Could you check a few things on this model? Use its own coordinates, in mm. A direction names the side the tool comes from. Coordinates: 2 decimals unless noted, no trailing zeros. Order: outer loops, then holes, each group sorted by start corner. A loop starts at its lowest first (then second) coordinate and runs counter-clockwise, first axis right, second up. Notation, with made-up numbers: M 48,17.25 L 74,17.25 A30 cw 74,43.25 Z; hole C 68.5,32.5 d8. An arc over 180 degrees is marked long. Put each result on its own line as item: value. Start each with the question number.
```python
from build123d import *

# Parameters (mm, degrees)
BOSS_EXTRUDE1_DEPTH = 5


with BuildPart() as part:
    # Sketch1 → Boss-Extrude1 (new body)
    with BuildSketch(Plane.XY):
        Polygon((25, 127.5), (20, 127.5), (20, 147.5), (25, 147.5), (25, 165), (32.5, 165), (32.5, 170), (47.5, 170), (47.5, 165), (55, 165), (55, 40), (47.5, 40), (47.5, 35), (32.5, 35), (32.5, 40), (25, 40), (25, 57.5), (20, 57.5), (20, 77.5), (25, 77.5), (25, 92.5), (20, 92.5), (20, 112.5), (25, 112.5), align=None)
    extrude(amount=-BOSS_EXTRUDE1_DEPTH)


solid = part.part
```
Item 1: For faces 5 (the flat face through (25, 85, -2)), 6 (the flat face through (25, 49, -2)), 7 (the flat face through (32.5, 167, -2)), 8 (the flat face through (47.5, 168, -2)), which set-ups out of +Z, -Z, +X, -X, +Y, -Y let a thin tool reach every point of the face, with its end or its side?
Item 2: If we section it at C-C on x = 52: Write out the boundary of the cut face in (y, z), then the cut area to 3 significant figures.
Item 3: If we section it at A-A on x = 23: Write out the boundary of the cut face in (y, z), then the cut area to 3 significant figures.
Item 4: I need wall thicknesses on probe 1 along X at (y, z) = (114, -1.2); probe 2 along Y at (x, z) = (53.5, -4.55). Which ranges of each line are inside material? Lowest first, please.
Item 5: If we section it at D-D on y = 79: Write out the boundary of the cut face in (x, z).
Item 6: For pin 1 Ø2.5 at (y, z) = (46, -3) entering from -X; pin 2 Ø1.5 at (y, z) = (38.5, -3) entering from -X; pin 3 Ø2.5 at (x, z) = (23, -2) entering from +Y; pin 4 Ø2 at (x, y) = (26, 123) entering from +Z, each with a flat end and sliding along its axis, tell me the tip position at first contact or that it passes through.
Item 7: If we mould it in two halves opening along Y, with no side actions, what happens to faces 1 (the flat face through (38, 103, -5)), 2 (the flat face through (29, 165, -2)), 3 (the flat face through (40, 35, -2)), 4 (the flat face through (22, 112.5, -2))? For each: released by +Y, released by -Y, zero draft, split by the parting line, or undercut.
Item 8: If we section it at B-B on z = -1.7: Write out the boundary of the cut face in (x, y).
Geometry check:
1. face 5: +Z, -Z, -X
1. face 6: +Z, -Z, -X, -Y
1. face 7: +Z, -Z, -X, +Y
1. face 8: +Z, -Z, +X, +Y
2. outline: M 40,-5 L 165,-5 L 165,0 L 40,0 Z
2. area: 625 mm²
3. outline: M 57.5,-5 L 77.5,-5 L 77.5,0 L 57.5,0 Z; M 92.5,-5 L 112.5,-5 L 112.5,0 L 92.5,0 Z; M 127.5,-5 L 147.5,-5 L 147.5,0 L 127.5,0 Z
3. area: 300 mm²
4. probe 1: x = 25 to 55
4. probe 2: y = 40 to 165
5. outline: M 25,-5 L 55,-5 L 55,0 L 25,0 Z
6. pin 1: stops at x = 25
6. pin 2: stops at x = 32.5
6. pin 3: stops at y = 147.5
6. pin 4: stops at z = 0
7. face 1: zero draft
7. face 2: released by +Y
7. face 3: released by -Y
7. face 4: undercut
8. outline: M 20,57.5 L 25,57.5 L 25,40 L 32.5,40 L 32.5,35 L 47.5,35 L 47.5,40 L 55,40 L 55,165 L 47.5,165 L 47.5,170 L 32.5,170 L 32.5,165 L 25,165 L 25,147.5 L 20,147.5 L 20,127.5 L 25,127.5 L 25,112.5 L 20,112.5 L 20,92.5 L 25,92.5 L 25,77.5 L 20,77.5 Z
